Build history of the part. All positions in model axes, mm. Coordinates: 2 decimals unless noted, no trailing zeros. Loops run counter-clockwise (first coordinate to the right, second up) from the corner with the lowest first, then second, coordinate; pieces in that order, holes last. Notation, with made-up numbers: (50.5, 62.25) - (67.5, 62.25) arc R27 ccw to (67.5, 90.25) - close; hole circle Ø7 at (77, 20). An arc over 180 degrees is marked (long way). One line per item, written item: value.
```python
from build123d import *

# Parameters (mm, degrees)
SKETCH2_R           = 4.05
SKETCH2_R_2         = 2
BOSS_EXTRUDE1_DEPTH = 10


with BuildPart() as part:
    # Sketch2 → Boss-Extrude1 (new body)
    with BuildSketch(Plane.XY):
        with BuildLine():
            Line((-52.525602652, 39.073613719), (55.40832582, 23.904489319))
            Line((55.40832582, 23.904489319), (88.545070057, 37.292603029))
            ThreePointArc((88.545070057, 37.292603029), (113.24947567, 26.806204997), (102.763077638, 2.101799383))
            Line((102.763077638, 2.101799383), (56.40388491, -16.628530288))
            Line((56.40388491, -16.628530288), (-52.525602652, -1.319489182))
            Line((-52.525602652, -1.319489182), (-84.855091861, -14.38145069))
            ThreePointArc((-84.855091861, -14.38145069), (-109.23231099, -4.033935081), (-98.88479538, 20.343284048))
            Line((-98.88479538, 20.343284048), (-52.525602652, 39.073613719))
        make_face()
        with Locations((-91.869943621, 2.980916679)):
            Circle(SKETCH2_R, mode=Mode.SUBTRACT)
        with Locations((95.654073847, 19.697201206)):
            Circle(SKETCH2_R, mode=Mode.SUBTRACT)
        with Locations((-52.525602652, 33.073613719)):
            Circle(SKETCH2_R_2, mode=Mode.SUBTRACT)
        with Locations((55.555695905, 17.904489319)):
            Circle(SKETCH2_R_2, mode=Mode.SUBTRACT)
        with Locations((-52.525602652, 4.680510818)):
            Circle(SKETCH2_R_2, mode=Mode.SUBTRACT)
        with Locations((56.256514825, -10.628530288)):
            Circle(SKETCH2_R_2, mode=Mode.SUBTRACT)
        with BuildLine():
            Line((-33.124360513, 22.209360939), (-11.338463, 19.147552718))
            ThreePointArc((-11.338463, 19.147552718), (-6.231893194, 12.3709057), (-13.008540212, 7.264335893))
            Line((-13.008540212, 7.264335893), (-34.794437724, 10.326144114))
            ThreePointArc((-34.794437724, 10.326144114), (-39.901007531, 17.102791132), (-33.124360513, 22.209360939))
        make_face(mode=Mode.SUBTRACT)
        with BuildLine():
            Line((-78.505415838, 13.773210112), (-67.379209583, 18.268489233))
            ThreePointArc((-67.379209583, 18.268489233), (-60.870257343, 15.505602928), (-63.633143649, 8.996650688))
            Line((-63.633143649, 8.996650688), (-74.759349904, 4.501371567))
            ThreePointArc((-74.759349904, 4.501371567), (-81.268302144, 7.264257873), (-78.505415838, 13.773210112))
        make_face(mode=Mode.SUBTRACT)
        with BuildLine():
            Line((67.013646361, 13.518391096), (78.139852616, 18.013670217))
            ThreePointArc((78.139852616, 18.013670217), (84.648804856, 15.250783911), (81.88591855, 8.741831672))
            Line((81.88591855, 8.741831672), (70.759712296, 4.246552551))
            ThreePointArc((70.759712296, 4.246552551), (64.250760056, 7.009438856), (67.013646361, 13.518391096))
        make_face(mode=Mode.SUBTRACT)
        with BuildLine():
            Line((16.389042924, 15.250705891), (38.174940437, 12.18889767))
            ThreePointArc((38.174940437, 12.18889767), (43.281510244, 5.412250652), (36.504863225, 0.305680845))
            Line((36.504863225, 0.305680845), (14.718965713, 3.367489066))
            ThreePointArc((14.718965713, 3.367489066), (9.612395906, 10.144136084), (16.389042924, 15.250705891))
        make_face(mode=Mode.SUBTRACT)
    extrude(amount=BOSS_EXTRUDE1_DEPTH)


solid = part.part
```
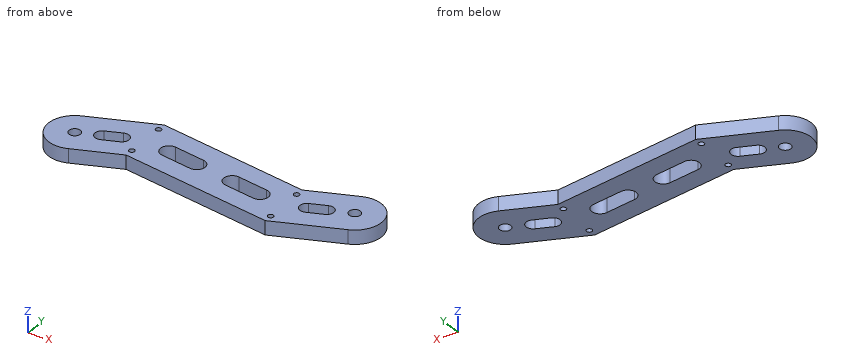
Item 1: Cut at B-B, the plane y = -5. Write the cut outline in (x, z), then the cut area to 3 significant figures.
Check result:
outline: (-108.81, 0) - (-61.64, 0) - (-61.64, 10) - (-108.81, 10) - close; (-26.34, 0) - (85.19, 0) - (85.19, 10) - (-26.34, 10) - close
area: 1,590 mm^2
Item 2: Cut at C-C, the plane z = 8.5. Give the number of separate pieces and of enclosed holes in the cut face, then the cut area to 3 significant figures.
Check result:
separate pieces: 1
enclosed holes: 10
area: 7,410 mm^2
Item 3: Probe probe 1 along Y at (x, z) = (-51, 3); probe 2 along Y at (x, z) = (-70.5, 8); probe 3 along Y at (x, z) = (22, 2.25). List the from-to ranges inside material, lowest first. Write a range as from..to.
Check result:
probe 1: y = -1.53..3.39, 5.97..31.78, 34.37..38.86
probe 2: y = -8.58..6.22, 17.01..31.81
probe 3: y = -11.79..2.34, 14.46..28.6
Item 4: Cut at D-D, the plane x = 3. Write the cut outline in (y, z).
Check result:
outline: (-9.12, 0) - (31.27, 0) - (31.27, 10) - (-9.12, 10) - close
Item 5: Cut at A-A, the plane x = 94.5. Write the cut outline in (y, z).
Check result:
outline: (-1.24, 0) - (15.82, 0) - (15.82, 10) - (-1.24, 10) - close; (23.58, 0) - (38.64, 0) - (38.64, 10) - (23.58, 10) - close
Item 6: Drop flat-ended pins along their axis: P1, Ø6, axis at x = 50, z = 9, coming from the -Y side; P2, Ø6, axis at y = 16.5, z = 8.5, coming from the +X side; P3, Ø1.5, axis at x = -7, z = 6, coming from the +Y side. Give the stop position or say it passes through.
Check result:
P1: stops at y = -16.15
P2: stops at x = 114.63
P3: stops at y = 32.78
